```python
from build123d import *

# Parameters (mm, degrees)
SKETCH_1_W          = 155.4
SKETCH_1_H          = 42
EXTRUDE_1_DEPTH     = 2.5
SKETCH_2_W          = 153.4
SKETCH_2_H          = 40
CUT_EXTRUDE_1_DEPTH = 0.5
SKETCH_3_W          = 1
SKETCH_3_H          = 6.2
SKETCH_3_W_2        = 6.2
SKETCH_3_H_2        = 1
CUT_EXTRUDE_2_DEPTH = 81.526641554
SKETCH_4_W          = 2
SKETCH_4_H          = 6.2
SKETCH_4_W_2        = 6.2
SKETCH_4_H_2        = 1.5
SKETCH_4_W_3        = 1.5
EXTRUDE_2_DEPTH     = 3
EXTRUDE_3_DEPTH     = 6.2
EXTRUDE_4_DEPTH     = 6.2


with BuildPart() as part:
    # Эскиз1 → Бобышка-Вытянуть1 (new body)
    with BuildSketch(Plane(origin=(0, 0, 0), x_dir=(1, 0, 0), z_dir=(0, 1, 0))):
        Rectangle(SKETCH_1_W, SKETCH_1_H)
    extrude(amount=EXTRUDE_1_DEPTH)

    # Эскиз2 → Вырез-Вытянуть1 (cut)
    with BuildSketch(Plane(origin=(0, 2.5, 0), x_dir=(1, 0, 0), z_dir=(0, 1, 0))):
        Rectangle(SKETCH_2_W, SKETCH_2_H)
    extrude(amount=-CUT_EXTRUDE_1_DEPTH, mode=Mode.SUBTRACT)

    # Эскиз3 → Вырез-Вытянуть2 (cut, through all)
    with BuildSketch(Plane(origin=(0, 2.5, 0), x_dir=(1, 0, 0), z_dir=(0, 1, 0))):
        with Locations((-77.2, 0)):
            Rectangle(SKETCH_3_W, SKETCH_3_H)
        with Locations((0, 20.5)):
            Rectangle(SKETCH_3_W_2, SKETCH_3_H_2)
        with Locations((0, -20.5)):
            Rectangle(SKETCH_3_W_2, SKETCH_3_H_2)
        with Locations((77.2, 0)):
            Rectangle(SKETCH_3_W, SKETCH_3_H)
    extrude(amount=-CUT_EXTRUDE_2_DEPTH, mode=Mode.SUBTRACT)

    # Эскиз4 → Бобышка-Вытянуть2 (add)
    with BuildSketch(Plane.XZ):
        with Locations((-75.7, 0)):
            Rectangle(SKETCH_4_W, SKETCH_4_H)
        with Locations((0, 19.25)):
            Rectangle(SKETCH_4_W_2, SKETCH_4_H_2)
        with Locations((0, -19.25)):
            Rectangle(SKETCH_4_W_2, SKETCH_4_H_2)
        with Locations((75.95, 0)):
            Rectangle(SKETCH_4_W_3, SKETCH_4_H)
    extrude(amount=EXTRUDE_2_DEPTH)

    # Эскиз6 → Бобышка-Вытянуть3 (add)
    with BuildSketch(Plane.XY.offset(3.1)):
        Polygon((-76.7, -3), (-77.2, -2.5), (-77.2, -1.5), (-76.6, -1.5), (-76.6, -3), align=None)
    extrude_3 = extrude(amount=-EXTRUDE_3_DEPTH)

    # Зеркальное отражение1: Бобышка-Вытянуть3 across plane
    add(extrude_3.mirror(Plane(origin=(0, 0, 0), x_dir=(0, 0, 1), z_dir=(1, 0, 0))))

    # Эскиз8 → Бобышка-Вытянуть4 (add)
    with BuildSketch(Plane(origin=(3.1, 0, 0), x_dir=(0, 0, -1), z_dir=(1, 0, 0))):
        Polygon((-20, -3), (-20.5, -2.5), (-20.5, -1.5), (-19.9, -1.5), (-19.9, -3), align=None)
    extrude_4 = extrude(amount=-EXTRUDE_4_DEPTH)

    # Зеркальное отражение2: Бобышка-Вытянуть4 across plane
    add(extrude_4.mirror(Plane.XY))


solid = part.part
```
Geometry check sheet. Reference: the model listing, model coordinates, mm. A direction names the side the tool comes from. Coordinates: 2 decimals unless noted, no trailing zeros. Write each loop counter-clockwise with the first axis right and the second up, starting at its lowest first coordinate (ties: lowest second). Pieces come first, ordered by that corner, then holes. Notation, with made-up numbers: M 16.25,35 L 34.25,35 A15 ccw 34.25,58 Z; hole C 60.5,37.25 d2. An arc over 180 degrees is marked long. One line per item, written item: value. Start each with the question number.
(1) Release check for a two-part mould opening along X. For faces 6 (the face through (-74.7, -1, 0)), 7 (the face through (77.7, 1, -12)), 8 (the face through (-76.7, 0, 0)), 9 (the face through (0, -1, -18.5)) record: released by +X, released by -X, zero draft, split by the parting line, or undercut.
(2) Sectioned sample at A-A, the plane z = 14. Enter the section's corners in (x, y), and give its area (3 significant figures).
(3) Scan lines: line 1 along Z through (x, y) = (-54.5, 2.1); line 2 along X through (y, z) = (-0.65, 0); line 3 along Y through (x, z) = (37.5, 9). Record each from-to range of solid material in increasing order. Write a range as [from, to].
(4) Depth check by flat-ended pin: pin 1 (1.6 mm diameter, centred on y = -2, z = -19.5, fed in from +X); pin 2 (0.9 mm diameter, centred on x = -0.5, y = -2, fed in from -Z); pin 3 (3 mm diameter, centred on x = 43, z = -7, fed in from +Y). Enter the tip coordinate at first touch or a pass-through.
(5) Sectioned sample at B-B, the plane x = 50. Enter the section's corners in (y, z).
(6) Tool access check on faces 1 (the face through (0, 0, 20)), 2 (the face through (-76, -1, 3.1)), 3 (the face through (-76, -1, -3.1)), 4 (the face through (-1, 2, 0)), 5 (the face through (76.7, 0, 0)). Record the directions out of +Z, -Z, +X, -X, +Y, -Y that give a thin tool (end or side, any length) a straight path to the whole face; none if there is none.
(7) Sectioned sample at C-C, the plane z = 0. Enter the section's corners in (x, y).
Filled sheet:
1. face 6: undercut
1. face 7: released by +X
1. face 8: released by -X
1. face 9: zero draft
2. outline: M -77.7,0 L 77.7,0 L 77.7,2.5 L 76.7,2.5 L 76.7,2 L -76.7,2 L -76.7,2.5 L -77.7,2.5 Z
2. area: 312 mm²
3. line 1: [-21, -20], [20, 21]
3. line 2: [-76.7, -74.7], [75.2, 76.7]
3. line 3: [0, 2]
4. pin 1: x = 3.1
4. pin 2: z = -20.5
4. pin 3: y = 2
5. outline: M 0,-21 L 2.5,-21 L 2.5,-20 L 2,-20 L 2,20 L 2.5,20 L 2.5,21 L 0,21 Z
6. face 1: +Z, +Y
6. face 2: +Z, +X, -X, -Y
6. face 3: -Z, +X, -X, -Y
6. face 4: +Y
6. face 5: +X, +Y
7. outline: M -77.2,-2.5 L -76.7,-3 L -74.7,-3 L -74.7,0 L 75.2,0 L 75.2,-3 L 76.7,-3 L 77.2,-2.5 L 77.2,-1.5 L 76.7,-1.5 L 76.7,2 L -76.7,2 L -76.7,-1.5 L -77.2,-1.5 Z
